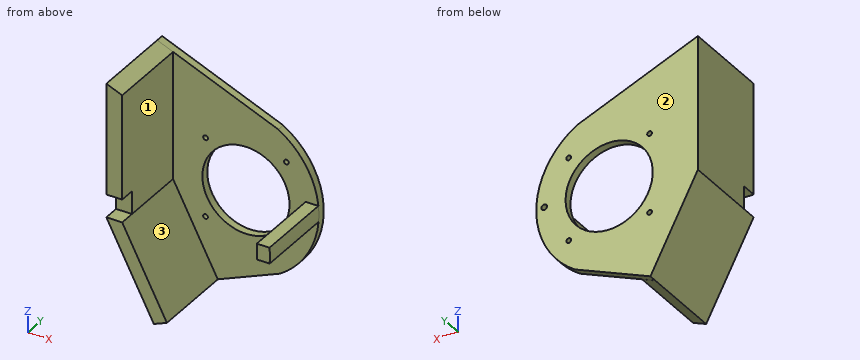
from build123d import *

# Parameters (mm, degrees)
SKETCH2_R           = 13.75
SKETCH2_R_2         = 0.75
BOSS_EXTRUDE1_DEPTH = 2.5
BOSS_EXTRUDE2_DEPTH = 26
SKETCH5_W           = 7.2
SKETCH5_H           = 21
BOSS_EXTRUDE5_DEPTH = 5
BOSS_EXTRUDE6_DEPTH = 25
SKETCH7_R           = 0.9
CUT_EXTRUDE1_DEPTH  = 10


with BuildPart() as part:
    # Sketch2 → Boss-Extrude1 (new body)
    with BuildSketch(Plane(origin=(0, 0, 0), x_dir=(1, 0, 0), z_dir=(0, 1, 0))):
        with BuildLine():
            Line((104.5, -77.2), (142.702591635, -61.456260882))
            ThreePointArc((142.702591635, -61.456260882), (155.478803114, -38.915145373), (143.235603671, -16.080138573))
            Line((143.235603671, -16.080138573), (119.48341621, -6.174842748))
            Line((119.48341621, -6.174842748), (104.5, -35))
            Line((104.5, -35), (104.5, -77.2))
        make_face()
        with Locations((132.490326991, -38.915145373)):
            Circle(SKETCH2_R, mode=Mode.SUBTRACT)
        with Locations((145.236491006, -25.853835985)):
            Circle(SKETCH2_R_2, mode=Mode.SUBTRACT)
        with Locations((119.744162977, -51.346164015)):
            Circle(SKETCH2_R_2, mode=Mode.SUBTRACT)
        with Locations((119.744162977, -26.484126731)):
            Circle(SKETCH2_R_2, mode=Mode.SUBTRACT)
        with Locations((145.236491006, -51.97645476)):
            Circle(SKETCH2_R_2, mode=Mode.SUBTRACT)
    extrude(amount=BOSS_EXTRUDE1_DEPTH)

    # Sketch3 → Boss-Extrude2 (add)
    with BuildSketch(Plane.XZ):
        Polygon((104.5, 42.2), (109.5, 42.2), (109.5, 75.139440959), (104.5, 77.2), align=None)
        Polygon((109.5, 35), (104.5, 35), (119.48341621, 6.174842748), (123.601295817, 7.871869559), align=None)
    extrude(amount=BOSS_EXTRUDE2_DEPTH)

    # Sketch5 → Boss-Extrude5 (add)
    with BuildSketch(Plane.ZY.offset(-104.5)):
        with Locations((38.6, -10.5)):
            Rectangle(SKETCH5_W, SKETCH5_H)
    extrude(amount=-BOSS_EXTRUDE5_DEPTH)

    # Sketch6 → Boss-Extrude6 (add)
    with BuildSketch(Plane.XZ):
        with BuildLine():
            Line((155.332558904, 41.415145373), (151.332558904, 41.415145373))
            Line((151.332558904, 41.415145373), (151.332558904, 36.415145373))
            Line((151.332558904, 36.415145373), (155.391548261, 36.415145373))
            ThreePointArc((155.391548261, 36.415145373), (155.478786901, 38.916522577), (155.332558904, 41.415145373))
        make_face()
    extrude(amount=BOSS_EXTRUDE6_DEPTH)

    # Sketch7 → Cut-Extrude1 (cut)
    with BuildSketch(Plane(origin=(0, 2.5, 0), x_dir=(1, 0, 0), z_dir=(0, 1, 0))):
        with Locations((152.978803114, -38.915145373)):
            Circle(SKETCH7_R)
    extrude(amount=-CUT_EXTRUDE1_DEPTH, mode=Mode.SUBTRACT)


solid = part.part
Geometry check sheet. Reference: the model listing, model coordinates, mm. Face numbers are marked on the shaded views. A direction names the side the tool comes from. Coordinates: 2 decimals unless noted, no trailing zeros. Loops run counter-clockwise (first coordinate to the right, second up) from the corner with the lowest first, then second, coordinate; pieces in that order, holes last. Notation, with made-up numbers: (-31, 77) - (-15, 77) arc R21 cw to (-15, 95) - close; hole circle Ø5 at (19, 68.5). An arc over 180 degrees is marked (long way). Use one line per item in the form item = value. Start each with the question number.
Item 1: Gauge pin test, flat ends, axial feed: pin 1 (1.2 mm diameter, centred on x = 119.74, z = 26.48, fed in from -Y) (3 decimals); pin 2 (5 mm diameter, centred on y = -11, z = 28.5, fed in from +X); pin 3 (4 mm diameter, centred on y = -5.5, z = 35, fed in from +X); pin 4 (1.5 mm diameter, centred on x = 107, z = 40, fed in from -Y). Record the tip position at first contact, or that the pin passes through.
Item 2: Tool access check on the marked faces 1, 2 and 3. Record the directions out of +Z, -Z, +X, -X, +Y, -Y that give a thin tool (end or side, any length) a straight path to the whole face; none if there is none.
Item 3: Section check A-A, the plane y = -22.5. Enter the section's corners in (x, z).
Item 4: Section check B-B, the plane z = 43.5. Enter the section's corners in (x, y).
Item 5: Section check C-C, the plane y = -2.25. Enter the section's corners in (x, z).
Item 6: Thickness scan on probe 1 along X at (y, z) = (-19.25, 66); probe 2 along Y at (x, z) = (124.5, 15.5); probe 3 along Z at (x, y) = (132, 0.75). Record the ranges inside material, lowest first.
Computed:
q1.pin_1 = through
q1.pin_2 = 114.18
q1.pin_3 = 155.43
q1.pin_4 = -21
q2.face_1 = +Z, -Y
q2.face_2 = +Z, -Z, +X, -X, +Y
q2.face_3 = +Z, +X, -Y
q3.outline = (104.5, 35) - (119.48, 6.17) - (123.6, 7.87) - (109.5, 35) - close; (104.5, 42.2) - (109.5, 42.2) - (109.5, 75.14) - (104.5, 77.2) - close; (151.33, 36.42) - (155.39, 36.42) arc R26.83 ccw to (155.33, 41.42) - (151.33, 41.42) - close
q4.outline = (104.5, -26) - (109.5, -26) - (109.5, 0) - (119.53, 0) - (119.53, 2.5) - (104.5, 2.5) - close; (145.45, 0) - (155.03, 0) - (155.03, 2.5) - (145.45, 2.5) - close
q5.outline = (104.5, 35) - (119.48, 6.17) - (123.6, 7.87) - (109.5, 35) - (109.5, 75.14) - (104.5, 77.2) - close; (151.33, 36.42) - (155.39, 36.42) arc R26.83 ccw to (155.33, 41.42) - (151.33, 41.42) - close; hole circle Ø1.8 at (152.98, 38.92)
q6.probe_1 = 104.5 to 109.5
q6.probe_2 = 0 to 2.5
q6.probe_3 = 11.39 to 25.17, 52.66 to 65.87
